from build123d import *

# Parameters (mm, degrees)
F0_R     = 19.05
F1_DEPTH = 219.075
F2_R     = 76.2
F3_DEPTH = 152.4


with BuildPart() as f1:
    # F0 (on Right) → F1 (new body, symmetric)
    with BuildSketch(Plane.YZ):
        Circle(F0_R)
    extrude(amount=F1_DEPTH, both=True)

    # F2 (on Right) → F3 (join, symmetric)
    with BuildSketch(Plane.YZ):
        Circle(F2_R)
    extrude(amount=F3_DEPTH, both=True)


solid = f1.part
Read the model definition and answer for the solid it produces. Units are mm, in the model's axes. A direction names the side the tool comes from. Give positions to 0.01 mm unless a question says otherwise; leave off trailing zeros. Write each loop counter-clockwise with the first axis right and the second up, starting at its lowest first coordinate (ties: lowest second). Pieces come first, ordered by that corner, then holes. Notation, with made-up numbers: (50, -18) - (57, -18) arc R24 cw to (57, 12) - close; hole circle Ø6 at (41, 68.5). An arc over 180 degrees is marked (long way). Answer in a Markdown table with one row per item. Add a question column.
Item 1: A tool of negligible diameter and unlimited length cuts with its end or side. For faces 1 (the face through (152.4, 16, -16)), 2 (the face through (-152.4, 16, -16)), 3 (the face through (2.134, -60.47, -46.367)), from which of +Z, -Z, +X, -X, +Y, -Y can it reach the whole face along a straight path? Write none if from no direction.
Item 2: Section C-C, the plane y = 33 is taken. Write down the section's boundary in (x, z), and give its area (3 significant figures).
Item 3: Section D-D, the plane z = 64 is taken. Write down the section's boundary in (x, y), and give its area (3 significant figures).
Item 4: Section A-A, the plane y = 0 is taken. Write down the section's boundary in (x, z) (3 decimals), and give its area (3 significant figures).
Item 5: Find the intervals of material crossed by L1, parallel to X at y = -65, z = 15; L2, parallel to Z at x = 107, y = 2.5; L3, parallel to Y at x = -110.5, z = -20.5, in increasing order.
Item 6: Flat-ended cylindrical pins translate along their axes: P1, Ø5, axis at x = 60, z = 9, coming from the -Y side; P2, Ø1.5, axis at y = -48.5, z = 2, coming from the +X side; P3, Ø2, axis at x = 133, z = -29.5, coming from the +Y side. Find the tip coordinate at first contact, or state that the pin passes through.
Recorded:
| question | item | result |
|---|---|---|
| 1 | face 1 | +X |
| 1 | face 2 | -X |
| 1 | face 3 | +X, -X |
| 2 | outline | (-152.4, -68.68) - (152.4, -68.68) - (152.4, 68.68) - (-152.4, 68.68) - close |
| 2 | area | 41,900 mm2 |
| 3 | outline | (-152.4, -41.36) - (152.4, -41.36) - (152.4, 41.36) - (-152.4, 41.36) - close |
| 3 | area | 25,200 mm2 |
| 4 | outline | (-219.075, -19.05) - (-152.4, -19.05) - (-152.4, -76.2) - (152.4, -76.2) - (152.4, -19.05) - (219.075, -19.05) - (219.075, 19.05) - (152.4, 19.05) - (152.4, 76.2) - (-152.4, 76.2) - (-152.4, 19.05) - (-219.075, 19.05) - close |
| 4 | area | 51,500 mm2 |
| 5 | L1 | x = -152.4 to 152.4 |
| 5 | L2 | z = -76.16 to 76.16 |
| 5 | L3 | y = -73.39 to 73.39 |
| 6 | P1 | stops at y = -75.92 |
| 6 | P2 | stops at x = 152.4 |
| 6 | P3 | stops at y = 70.67 |
